```python
from build123d import *

# Parameters (mm, degrees)
SKETCH_R        = 17.5
SKETCH_R_2      = 4
PAD_DEPTH       = 2
SKETCH001_R     = 15
SKETCH001_R_2   = 13.5
PAD001_DEPTH    = 3
SKETCH002_R     = 3
POCKET_DEPTH    = 5
SKETCH004_R     = 2.5
POCKET001_DEPTH = 2.001


with BuildPart() as part:
    # Sketch → Pad (new body)
    with BuildSketch(Plane.XY):
        Circle(SKETCH_R)
        Circle(SKETCH_R_2, mode=Mode.SUBTRACT)
    extrude(amount=PAD_DEPTH)

    # Sketch001 (on Face4 of Pad) → Pad001 (join)
    with BuildSketch(Plane.XY.offset(2)):
        Circle(SKETCH001_R)
        Circle(SKETCH001_R_2, mode=Mode.SUBTRACT)
    extrude(amount=PAD001_DEPTH)

    # Sketch002 (on Face2 of Pad001) → Pocket (cut)
    with BuildSketch(Plane(origin=(0, 0, 0), x_dir=(1, 0, 0), z_dir=(0, 0, -1))):
        with Locations((-10, 0)):
            Circle(SKETCH002_R)
        with Locations((10, 0)):
            Circle(SKETCH002_R)
    extrude(amount=-POCKET_DEPTH, mode=Mode.SUBTRACT)

    # Sketch004 (on Face8 of Pocket) → Pocket001 (cut, through all)
    with BuildSketch(Plane.XY.offset(2)):
        with Locations((3.762222, -10.336619)):
            Circle(SKETCH004_R)
        with Locations((-3.762222, -10.336619)):
            Circle(SKETCH004_R)
        with Locations((3.762222, 10.336619)):
            Circle(SKETCH004_R)
        with Locations((-3.762222, 10.336619)):
            Circle(SKETCH004_R)
    extrude(amount=-POCKET001_DEPTH, mode=Mode.SUBTRACT)


solid = part.part
```
Geometry check sheet. Reference: the model listing, model coordinates, mm. A direction names the side the tool comes from. Coordinates: 2 decimals unless noted, no trailing zeros. Write each loop counter-clockwise with the first axis right and the second up, starting at its lowest first coordinate (ties: lowest second). Pieces come first, ordered by that corner, then holes. Notation, with made-up numbers: (-11.75, 53) -> (10.25, 53) arc R13 ccw to (10.25, 66) -> close; hole circle Ø2 at (18.25, -14). An arc over 180 degrees is marked (long way). Use CSV: the item, a comma, the result in double quotes. Start each with the question number.
Item 1: Cross-section at C-C, the plane y = 9.5. Record the cut outline in (x, z).
Item 2: Set-up check for faces 1 (the flat face through (13, 8, 2)), 2 (the cylindrical face through (3.437, -7.858, 1.014)): record each of +Z, -Z, +X, -X, +Y, -Y from which the full face is reachable in a straight line by a thin tool's end or side.
Item 3: Cross-section at D-D, the plane z = 3. Record the cut outline in (x, y), plus the area to 3 significant figures.
Item 4: Cross-section at B-B, the plane x = 0. Record the cut outline in (y, z).
Item 5: Depth check by flat-ended pin: pin 1 Ø8 at (x, y) = (3.76, 10.34) entering from -Z; pin 2 Ø17.5 at (x, y) = (-2, 3.5) entering from +Z; pin 3 Ø1 at (x, z) = (2, 1) entering from -Y; pin 4 Ø1 at (y, z) = (-3, 1.5) entering from +X. Enter the tip coordinate at first touch or a pass-through.
Item 6: Cross-section at A-A, the plane y = 0. Record the cut outline in (x, z).
Item 7: Thickness scan on line 1 (Y direction, x = -3, z = 1.3); line 2 (Y direction, x = 0, z = 1.5); line 3 (Z direction, x = -7, y = -3). Record the ranges inside material, lowest first.
Item 8: Mould release check, pull along X, two halves, no side actions. Record for faces 3 (the flat face through (-11.18, 7.85, 5)), 4 (the flat face through (-3, -3, 2)), 5 (the cylindrical face through (-14.985, 0.66, 3.479)): released by +X, released by -X, zero draft, split by the parting line, or undercut.
Answers:
1,outline,"(-14.7, 0) -> (-6.12, 0) -> (-6.12, 2) -> (-9.59, 2) -> (-9.59, 5) -> (-11.61, 5) -> (-11.61, 2) -> (-14.7, 2) -> close; (-1.41, 0) -> (1.41, 0) -> (1.41, 2) -> (-1.41, 2) -> close; (6.12, 0) -> (14.7, 0) -> (14.7, 2) -> (11.61, 2) -> (11.61, 5) -> (9.59, 5) -> (9.59, 2) -> (6.12, 2) -> close"
2,face 1,"+Z"
2,face 2,"+Z, -Z"
3,outline,"circle Ø30 at (0, 0); hole circle Ø27 at (0, 0)"
3,area,"134 mm^2"
4,outline,"(-17.5, 0) -> (-4, 0) -> (-4, 2) -> (-13.5, 2) -> (-13.5, 5) -> (-15, 5) -> (-15, 2) -> (-17.5, 2) -> close; (4, 0) -> (17.5, 0) -> (17.5, 2) -> (15, 2) -> (15, 5) -> (13.5, 5) -> (13.5, 2) -> (4, 2) -> close"
5,pin 1,"z = 0"
5,pin 2,"z = 2"
5,pin 3,"y = -17.44"
5,pin 4,"x = 17.32"
6,outline,"(-17.5, 0) -> (-13, 0) -> (-13, 2) -> (-13.5, 2) -> (-13.5, 5) -> (-15, 5) -> (-15, 2) -> (-17.5, 2) -> close; (-7, 0) -> (-4, 0) -> (-4, 2) -> (-7, 2) -> close; (4, 0) -> (7, 0) -> (7, 2) -> (4, 2) -> close; (13, 0) -> (17.5, 0) -> (17.5, 2) -> (15, 2) -> (15, 5) -> (13.5, 5) -> (13.5, 2) -> (13, 2) -> close"
7,line 1,"-17.24 to -12.72, -7.96 to -2.65, 2.65 to 7.96, 12.72 to 17.24"
7,line 2,"-17.5 to -4, 4 to 17.5"
7,line 3,"0 to 2"
8,face 3,"zero draft"
8,face 4,"undercut"
8,face 5,"split by the parting line"
